For this review, take the finished solid that the model builds, in its own axes (mm). Face numbers are marked on the shaded views. A direction names the side the tool comes from. Give positions to 0.01 mm unless a question says otherwise; leave off trailing zeros. Write each loop counter-clockwise with the first axis right and the second up, starting at its lowest first coordinate (ties: lowest second). Pieces come first, ordered by that corner, then holes.
Q1. We need section A-A (z = -6). Write out the cut boundary in (x, y).
Q2. Insertion check: P1, Ø2.5, axis at x = -5.5, y = -1.5, coming from the +Z side; P2, Ø1.1, axis at x = -8.5, z = 2, coming from the -Y side; P3, Ø0.8, axis at x = -8.5, z = 1, coming from the +Y side. Each pin has a flat end and moves straight along its axis. Give the tip position at first contact, or say it passes through.
Q3. For line 1 (Z direction, x = -5, y = -0.75); line 2 (Y direction, x = -6.5, z = -0.25); line 3 (Z direction, x = -6.75, y = 2.5), list the stretches that pass through material, from the lowest coordinate up.
Q4. We need section B-B (x = -6). Write out the cut boundary in (y, z).
Q5. We need section C-C (y = 3). Write out the cut boundary in (x, z), then the cut area to 3 significant figures.
Q6. We need section D-D (x = -11). Write out the cut boundary in (y, z).
Q7. Machinability: for the marked faces 1 and 2, which of the approach directions +Z, -Z, +X, -X, +Y, -Y give a long, thin tool a straight path to every point of the face, cutting with its end or side? Answer none if there is none.
Autodesk Inventor part; units mm, degrees
ref_plane "YZ Plane" through (0, 0, 0) normal (1, 0, 0) x (0, 1, 0)
ref_plane "XZ Plane" through (0, 0, 0) normal (0, 1, 0) x (-1, 0, 0)
ref_plane "XY Plane" through (0, 0, 0) normal (0, 0, 1) x (1, 0, 0)
sketch "Sketch1" plane through (0, 0, 0) normal (0, 1, 0) x (-1, 0, 0)
  line L0 (12, -12) -> (0, -12)
  line L1 (0, -12) -> (0, 0)
  line L2 (0, 0) -> (12, 0)
  line L3 (12, 0) -> (12, -12)
  circle A0 centre (6, -6) radius 3.4
  line L4 (12, 0) -> (0, -12) construction
  point P0 (6, -6)
  dimension "d0" = 12
  dimension "d1" = 12
  dimension "d4" = 6.8
extrude "Extrusion1" add sketch "Sketch1" against normal blind 3.25 contours L0 L1 L2 L3 | A0
extrude "Extrusion2" add sketch "Sketch1" along normal blind 4.8 contours A0
ref_plane "Work Plane1" through (-3, 0, 0) normal (1, 0, 0) x (0, 0, -1)
sketch "Sketch2" plane through (-3, 0, 0) normal (1, 0, 0) x (0, 0, -1)
  line L0 (12, -3.25) -> (0, -3.25)
  line L1 (12, -2.55) -> (16, -2.55)
  line L2 (16, -2.55) -> (16, -2.25)
  line L3 (16, -2.25) -> (12, -2.25)
  line L4 (12, -2.25) -> (12, -2.55)
  line L5 (12, 0) -> (12, -3.25)
  point P0 (0, 0)
  dimension "d8" = 4
  dimension "d9" = 0.3
  dimension "d10" = 0.7
extrude "Extrusion3" add sketch "Sketch2" against normal blind 1
ref_plane "Work Plane2" through (-6, 0, 0) normal (1, 0, 0) x (0, 0, -1)
ref_plane "Work Plane3" through (0, 0, -6) normal (0, 0, -1) x (-1, 0, 0)
mirror "Mirror1" about plane through (-6, 0, 0) normal (1, 0, 0) of "Extrusion3"
mirror "Mirror2" about plane through (0, 0, -6) normal (0, 0, -1) of "Extrusion3", "Mirror1"
properties part number "Button"
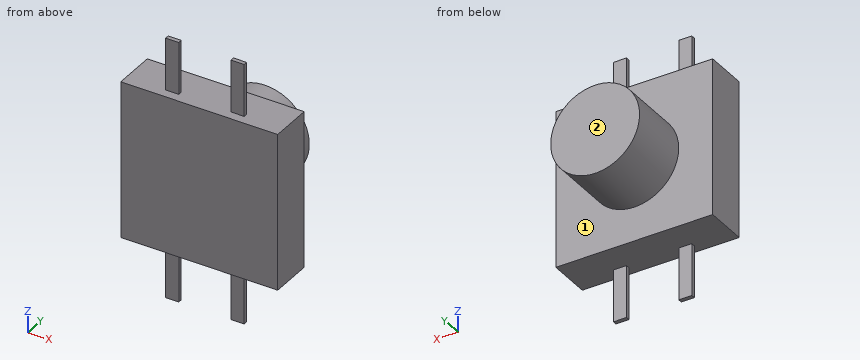
Computed:
1. outline: (-12, -3.25) - (0, -3.25) - (0, 0) - (-2.6, 0) - (-2.6, 4.8) - (-9.4, 4.8) - (-9.4, 0) - (-12, 0) - close
2. P1: stops at z = 0
2. P2: stops at y = -2.55
2. P3: stops at y = -2.25
3. line 1: z = -12 to 0
3. line 2: y = -3.25 to 0
3. line 3: z = -9.32 to -2.68
4. outline: (-3.25, -12) - (0, -12) - (0, -9.4) - (4.8, -9.4) - (4.8, -2.6) - (0, -2.6) - (0, 0) - (-3.25, 0) - close
5. outline: circle Ø6.8 at (-6, -6)
5. area: 36.3 mm2
6. outline: (-3.25, -12) - (0, -12) - (0, 0) - (-3.25, 0) - close
7. face 1: +Y
7. face 2: +Z, -Z, +X, -X, +Y
